Autodesk Inventor part; units mm, degrees
ref_plane "YZ Plane" through (0, 0, 0) normal (1, 0, 0) x (0, 1, 0)
ref_plane "XZ Plane" through (0, 0, 0) normal (0, 1, 0) x (-1, 0, 0)
ref_plane "XY Plane" through (0, 0, 0) normal (0, 0, 1) x (1, 0, 0)
sketch "Sketch1" plane through (0, 0, 0) normal (0, 0, 1) x (1, 0, 0)
  line L0 (0, 30) -> (20, 30)
  line L1 (20, 30) -> (20, 0)
  line L2 (20, 0) -> (0, 0)
  line L3 (0, 0) -> (0, 30)
  circle A0 centre (10, 15) radius 2.5
  dimension "d0" = 30
  dimension "d1" = 20
  dimension "d5" = 10
  dimension "d6" = 15
  dimension "d7" = 5
extrude "Extrusion2" add sketch "Sketch1" along normal blind 25
sketch "Sketch4" plane through (0, 0, 25) normal (0, 0, 1) x (1, 0, 0)
  line L0 (0, 0) -> (20, 0)
  line L1 (0, 0) -> (-50, 0)
  line L2 (-50, 0) -> (-50, 12)
  line L3 (-50, 12) -> (0, 12)
  line L4 (0, 12) -> (0, 0)
  point P0 (0, 6)
  dimension "d13" = 12
  dimension "d14" = 50
extrude "Extrusion4" add sketch "Sketch4" against normal blind 100
sketch "Sketch5" plane through (0, 0, 0) normal (0, 0, -1) x (-1, 0, 0)
  line L0 (0, 0) -> (-20, 0)
  line L1 (-20, 0) -> (-20, 30)
  line L2 (0, 0) -> (-20, 0)
  line L3 (-20, 0) -> (-20, 30)
  line L4 (-20, 30) -> (0, 30)
  line L5 (0, 30) -> (0, 0)
  circle A0 centre (-10, 15) radius 2.5
  circle A1 centre (-10, 15) radius 4.5
  dimension "d17" = 9
extrude "Extrusion5" add sketch "Sketch5" along normal blind 75 contours L0 L1 L4 L5
properties part number "Touchscreen mount R v05"
Work out the finished part from the listing and answer in its coordinate system (mm). A direction names the side the tool comes from. Coordinates: 2 decimals unless noted, no trailing zeros. Loops run counter-clockwise (first coordinate to the right, second up) from the corner with the lowest first, then second, coordinate; pieces in that order, holes last. Notation, with made-up numbers: (-22, 40) -> (12, 40) arc R18 cw to (12, 61) -> close; hole circle Ø7 at (72, -37.5). An arc over 180 degrees is marked (long way). Write each question's results on one line, items separated by ' | '. Start each with the question number.
1) Find section B-B on z = -4. Determine the outline of the cut face in (x, y).
2) The mould has two halves that part along Y. Classify faces 4 (the flat face through (10, 30, -24)), 5 (the flat face through (-7, 9, -75)), 6 (the cylindrical face through (9.46, 17.44, 12.32)): pulls with the +Y half, pulls with the -Y half, needs draft (parallel to the pull), parting line crosses it, or undercut.
3) For faces 1 (the flat face through (-8, 9, 25)), 2 (the flat face through (-25, 12, -24)), 3 (the cylindrical face through (7.581, 11.206, -36.975)), determine the directions among +Z, -Z, +X, -X, +Y, -Y from which every point of the face is accessible in a straight line to the end or side of a thin tool.
4) Find section A-A on y = 15. Determine the outline of the cut face in (x, z).
5) Flat-ended cylindrical pins translate along their axes: P1, Ø8, axis at x = 10, y = 15, coming from the -Z side; P2, Ø5.5, axis at y = 17.5, z = -9.5, coming from the -X side. Find the tip coordinate at first contact, or state that the pin passes through.
6) Find section C-C on x = 10. Determine the outline of the cut face in (y, z).
7) Consider line 1 along X through (y, z) = (18.75, -17); line 2 along Y through (x, z) = (10, -40); line 3 along Y through (x, z) = (10, 10.75). Determine where each line is inside the solid, lowest interval first.
8) Find section D-D on y = 25.25. Determine the outline of the cut face in (x, z).
Response values:
1) outline: (-50, 0) -> (20, 0) -> (20, 30) -> (0, 30) -> (0, 12) -> (-50, 12) -> close; hole circle Ø9 at (10, 15)
2) face 4: pulls with the +Y half | face 5: needs draft | face 6: undercut
3) face 1: +Z, +X, -X, +Y, -Y | face 2: +Z, -Z, -X, +Y | face 3: -Z
4) outline: (0, -75) -> (5.5, -75) -> (5.5, 0) -> (7.5, 0) -> (7.5, 25) -> (0, 25) -> close; (12.5, 0) -> (14.5, 0) -> (14.5, -75) -> (20, -75) -> (20, 25) -> (12.5, 25) -> close
5) P1: stops at z = 0 | P2: stops at x = 0
6) outline: (0, -75) -> (10.5, -75) -> (10.5, 0) -> (12.5, 0) -> (12.5, 25) -> (0, 25) -> close; (17.5, 0) -> (19.5, 0) -> (19.5, -75) -> (30, -75) -> (30, 25) -> (17.5, 25) -> close
7) line 1: x = 0 to 7.51, 12.49 to 20 | line 2: y = 0 to 10.5, 19.5 to 30 | line 3: y = 0 to 12.5, 17.5 to 30
8) outline: (0, -75) -> (20, -75) -> (20, 25) -> (0, 25) -> close
